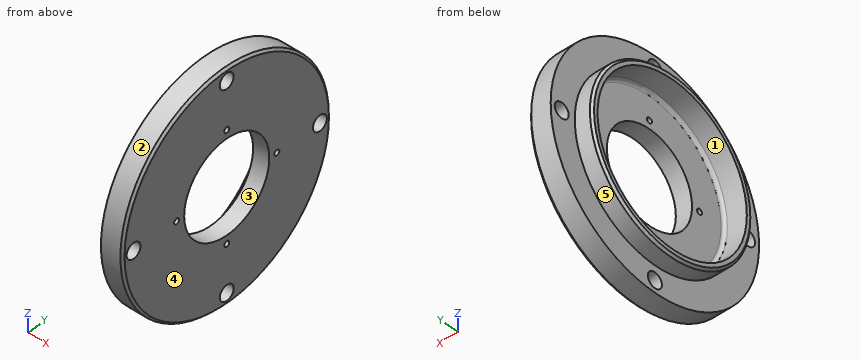
from build123d import *

# Parameters (mm, degrees)
F0_R     = 104
F1_DEPTH = 20
F2_R     = 80
F3_DEPTH = 16
F4_SIZE  = 2
F5_R     = 74.5
F6_DEPTH = 21
F7_R     = 3
F9_D     = 85
F11_D    = 5
F13_D    = 14


with BuildPart() as f1:
    # F0 (on Right) → F1 (new body)
    with BuildSketch(Plane.YZ):
        Circle(F0_R)
    extrude(amount=F1_DEPTH)

    # F2 (on face) → F3 (join)
    with BuildSketch(Plane(origin=(0, 0, 0), x_dir=(0, -1, 0), z_dir=(-1, 0, 0))):
        Circle(F2_R)
    extrude(amount=F3_DEPTH)

    # F4
    f4_edges = [f1.edges().sort_by_distance(p)[0] for p in [
        (-16, 80, 0),
        (20, -104, 0),
    ]]
    chamfer(f4_edges, length=F4_SIZE)

    # F5 (on face) → F6 (cut)
    with BuildSketch(Plane(origin=(-16, 0, 0), x_dir=(0, -1, 0), z_dir=(-1, 0, 0))):
        Circle(F5_R)
    extrude(amount=-F6_DEPTH, mode=Mode.SUBTRACT)

    # F7
    f7_edges = [f1.edges().sort_by_distance(p)[0] for p in [
        (5, 74.5, 0),
    ]]
    fillet(f7_edges, radius=F7_R)

    # F9 (through all)
    with Locations(Plane.YZ.offset(20)):
        with Locations((0, 0)):
            Hole(F9_D / 2)

    # F11 (through all)
    with Locations(Plane.YZ.offset(20)):
        with Locations((0, 50), (50, 0), (0, -50), (-50, 0)):
            Hole(F11_D / 2)

    # F13 (through all)
    with Locations(Plane.YZ.offset(20)):
        with Locations((0, 93), (93, 0), (0, -93), (-93, 0)):
            Hole(F13_D / 2)


solid = f1.part
Part model, mm, in its own coordinate system. Face numbers are marked on the shaded views. A direction names the side the tool comes from. Coordinates: 2 decimals unless noted, no trailing zeros. Loops run counter-clockwise (first coordinate to the right, second up) from the corner with the lowest first, then second, coordinate; pieces in that order, holes last. Notation, with made-up numbers: (-4.75, 54) - (29.25, 54) arc R20 ccw to (29.25, 66) - close; hole circle Ø10 at (48, 41.25). An arc over 180 degrees is marked (long way). Write each question's results on one line, items separated by ' | '. Start each with the question number.
Q1. Slice it at B-B on x = -3.5. Give the cut face in (y, z), and give its area (3 significant figures).
Q2. Which spindle directions (+Z, -Z, +X, -X, +Y, -Y) get a long thin tool onto all of the face, cutting with end or side? Do the marked faces 1 and 2. Say none if no direction does.
Q3. Drop flat-ended pins along their axis: pin 1 Ø1.5 at (y, z) = (7.5, -60) entering from -X; pin 2 Ø1.5 at (x, z) = (-3.5, 47) entering from +Y; pin 3 Ø2 at (x, y) = (-5.5, 25.5) entering from -Z. Give the stop position or say it passes through.
Q4. Probe line 1 along Z through (x, y) = (13.5, 0); line 2 along Z through (x, y) = (-7.5, 0); line 3 along X through (y, z) = (12.5, 44.5). List the from-to ranges inside material, lowest first.
Q5. Two-plate mould, pull along Z, no slides. Class the marked faces 3, 4 and 5: +Z half, -Z half, draft (parallel to the pull), parting line (faces both ways), or undercut.
Q6. Slice it at A-A on z = 0. Give the number of separate pieces and of enclosed holes in the cut face, and give its area (3 significant figures).
Answer:
1) outline: circle Ø160 at (0, 0); hole circle Ø149 at (0, 0) | area: 2,670 mm2
2) face 1: -X | face 2: +X, -X
3) pin 1: stops at x = 5 | pin 2: stops at y = 65.28 | pin 3: stops at z = -76.16
4) line 1: z = -104 to -100, -86 to -52.5, -47.5 to -42.5, 42.5 to 47.5, 52.5 to 86, 100 to 104 | line 2: z = -80 to -74.5, 74.5 to 80 | line 3: x = 5 to 20
5) face 3: undercut | face 4: draft | face 5: parting line
6) separate pieces: 6 | enclosed holes: 0 | area: 1,600 mm2
